Here's the drawing with two shaded views (mm, measured from the low corner). I have some questions. A direction names the side the tool comes from. Give positions to 0.01 mm unless a question says otherwise; leave off trailing zeros. Loops run counter-clockwise (first coordinate to the right, second up) from the corner with the lowest first, then second, coordinate; pieces in that order, holes last. Notation, with made-up numbers: (49, 14) - (64, 14) arc R25 ccw to (64, 30) - close; hole circle Ø5 at (-12, -30). An arc over 180 degrees is marked (long way). Answer as a JSON object with one key per item and string values. Group by question number.
Item 1: Suppose I cut it at B-B on x = 15. Write out the boundary of the cut face in (y, z).
Item 2: Will these pins go through, and if not, where does the flat tip stop? pin 1 (2.5 mm diameter, centred on x = 5, z = 15, fed in from -Y); pin 2 (5 mm diameter, centred on x = 15, z = 5, fed in from -Y); pin 3 (8 mm diameter, centred on x = 20, z = 19.5, fed in from +Y); pin 4 (1 mm diameter, centred on x = 14.5, y = 2, fed in from +Z).
Item 3: Please list where these lines run through material, in increasing order: L1, parallel to Z at x = 15, y = 0.65; L2, parallel to Z at x = 15, y = 2.2; L3, parallel to X at y = 1.6, z = 15.
Item 4: Suppose I cut it at C-C on y = 4. Write out the boundary of the cut face in (x, z).
Item 5: Which directions (+Z, -Z, +X, -X, +Y, -Y) give clear straight access to the entire face, cutting with the end or side of a thin tool? Please do the marked faces 1 and 2.
Item 6: Suppose I cut it at A-A on z = 15. Write out the boundary of the cut face in (x, y), and give its area (3 significant figures).
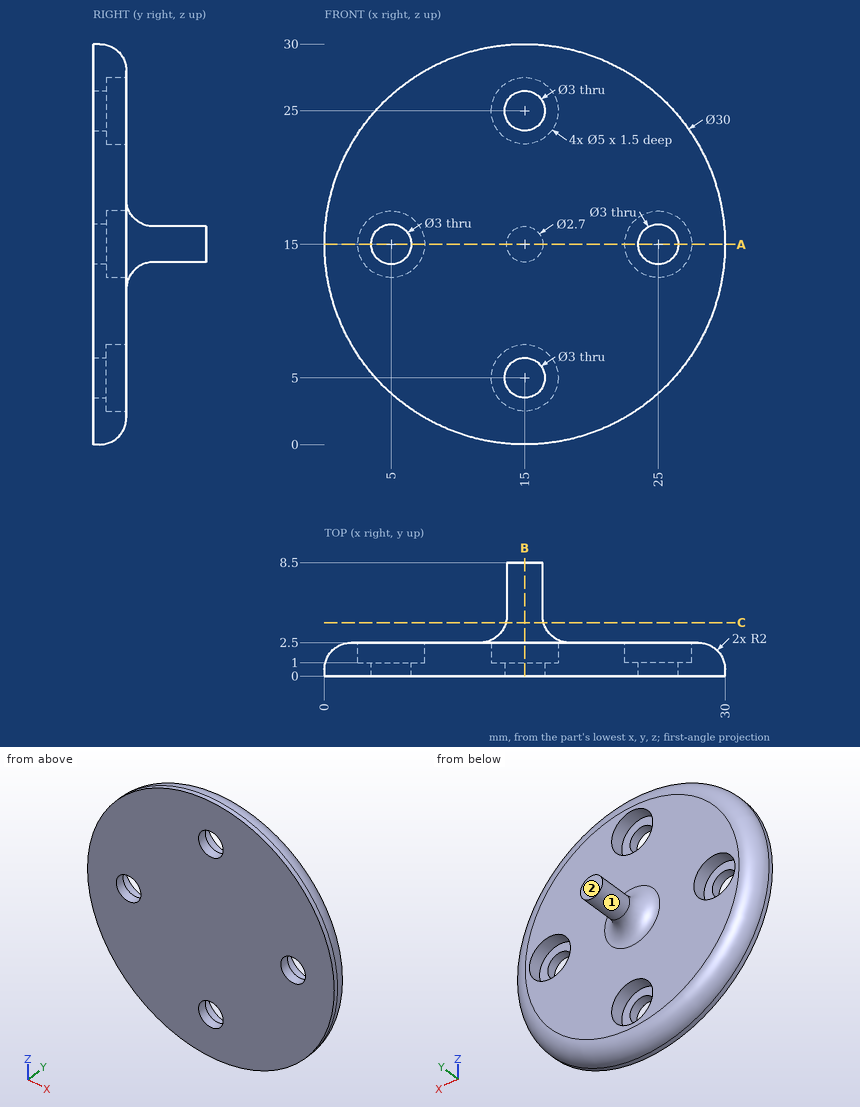
Worked out:
{
 "1": {"outline": "(0, 0) - (0.5, 0) arc R2 ccw to (2.5, 2) - (2.5, 2.5) - (1, 2.5) - (1, 3.5) - (0, 3.5) - close; (0, 6.5) - (1, 6.5) - (1, 7.5) - (2.5, 7.5) - (2.5, 11.65) arc R2 cw to (4.5, 13.65) - (8.5, 13.65) - (8.5, 16.35) - (4.5, 16.35) arc R2 cw to (2.5, 18.35) - (2.5, 22.5) - (1, 22.5) - (1, 23.5) - (0, 23.5) - close; (0, 26.5) - (1, 26.5) - (1, 27.5) - (2.5, 27.5) - (2.5, 28) arc R2 ccw to (0.5, 30) - (0, 30) - close"},
 "2": {"pin 1": "passes through", "pin 2": "stops at y = 0", "pin 3": "stops at y = 2.6", "pin 4": "stops at z = 29.72"},
 "3": {"L1": "z = 0.01 to 3.5, 6.5 to 23.5, 26.5 to 29.99", "L2": "z = 0.95 to 2.5, 7.5 to 22.5, 27.5 to 29.05", "L3": "x = 0.33 to 2.5, 7.5 to 22.5, 27.5 to 29.67"},
 "4": {"outline": "circle Ø2.83 at (15, 15)"},
 "5": {"face 1": "+Y", "face 2": "+Z, -Z, +X, -X, +Y"},
 "6": {"outline": "(0, 0) - (3.5, 0) - (3.5, 1) - (2.5, 1) - (2.5, 2.5) - (2, 2.5) arc R2 ccw to (0, 0.5) - close; (6.5, 0) - (23.5, 0) - (23.5, 1) - (22.5, 1) - (22.5, 2.5) - (18.35, 2.5) arc R2 cw to (16.35, 4.5) - (16.35, 8.5) - (13.65, 8.5) - (13.65, 4.5) arc R2 cw to (11.65, 2.5) - (7.5, 2.5) - (7.5, 1) - (6.5, 1) - close; (26.5, 0) - (30, 0) - (30, 0.5) arc R2 ccw to (28, 2.5) - (27.5, 2.5) - (27.5, 1) - (26.5, 1) - close", "area": "70.2 mm2"}
}
